```python
from build123d import *

# Parameters (mm, degrees)
BOSS_EXTRUDE2_DEPTH = 10
SKETCH6_R           = 5
CUT_EXTRUDE2_DEPTH  = 202.494416796


with BuildPart() as part:
    # Sketch5 → Boss-Extrude2 (new body)
    with BuildSketch(Plane.XY):
        Polygon((0, 0), (180, 0), (0, -90), align=None)
    extrude(amount=-BOSS_EXTRUDE2_DEPTH)

    # Sketch6 → Cut-Extrude2 (cut, through all)
    with BuildSketch(Plane.XY):
        with Locations((15, -20)):
            Circle(SKETCH6_R)
        with Locations((15, -60)):
            Circle(SKETCH6_R)
    extrude(amount=-CUT_EXTRUDE2_DEPTH, mode=Mode.SUBTRACT)


solid = part.part
```
Geometry check sheet. Reference: the model listing, model coordinates, mm. Coordinates: 2 decimals unless noted, no trailing zeros. Order: outer loops, then holes, each group sorted by start corner. A loop starts at its lowest first (then second) coordinate and runs counter-clockwise, first axis right, second up. Notation, with made-up numbers: M 5.5,49 L 11.5,49 A33 cw 11.5,84 Z; hole C 27,82.5 d9. An arc over 180 degrees is marked long. Answer as a JSON object with one key per item and string values.
Q1. Depth check by flat-ended pin: pin 1 Ø4 at (y, z) = (-55, -5) entering from +X; pin 2 Ø4 at (y, z) = (-19.5, -5) entering from -X; pin 3 Ø1.5 at (x, z) = (35.5, -1.5) entering from -Y (3 decimals); pin 4 Ø5 at (x, z) = (61.5, -4) entering from -Y. Enter the tip coordinate at first touch or a pass-through.
Results are:
{"pin 1": "stops at x = 74", "pin 2": "stops at x = 0", "pin 3": "stops at y = -72.625", "pin 4": "stops at y = -60.5"}
Q2. Release check for a two-part mould opening along Y. For faces 1 (the flat face through (51, -24, 0)), 2 (the cylindrical face through (18, -56, -5)), 3 (the flat face through (91.26, -44.37, -4.93)), 4 (the cylindrical face through (17.307, -24.436, -4.93)) record: released by +Y, released by -Y, zero draft, split by the parting line, or undercut.
Results are:
{"face 1": "zero draft", "face 2": "undercut", "face 3": "released by -Y", "face 4": "undercut"}
Q3. Cross-section at D-D on x = 160. Record the cut outline in (y, z).
Results are:
{"outline": "M -10,-10 L 0,-10 L 0,0 L -10,0 Z"}
Q4. Scan lines: line 1 (Y direction, x = 15, z = -4.5); line 2 (X direction, y = -22, z = -5.75); line 3 (X direction, y = -52, z = -7.5). Record each from-to range of solid material in increasing order.
Results are:
{"line 1": "y = -82.5 to -65, -55 to -25, -15 to 0", "line 2": "x = 0 to 10.42, 19.58 to 136", "line 3": "x = 0 to 76"}
Q5. Cross-section at A-A on y = -60. Record the cut outline in (x, z).
Results are:
{"outline": "M 0,-10 L 10,-10 L 10,0 L 0,0 Z; M 20,-10 L 60,-10 L 60,0 L 20,0 Z"}
Q6. Cross-section at C-C on y = -20. Record the cut outline in (x, z), and give its area (3 significant figures).
Results are:
{"outline": "M 0,-10 L 10,-10 L 10,0 L 0,0 Z; M 20,-10 L 140,-10 L 140,0 L 20,0 Z", "area": "1,300 mm²"}
Q7. Cross-section at B-B on z = -4.75. Record the cut outline in (x, y).
Results are:
{"outline": "M 0,-90 L 180,0 L 0,0 Z; hole C 15,-60 d10; hole C 15,-20 d10"}
